from build123d import *

# Parameters (mm, degrees)
SKETCH_1_R      = 1
EXTRUDE_1_DEPTH = 1
FILLET_1_R      = 2


with BuildPart() as part:
    # 草图1 → 凸台-拉伸1 (new body)
    with BuildSketch(Plane(origin=(0, 0, 0), x_dir=(1, 0, 0), z_dir=(0, 1, 0))):
        with BuildLine():
            Line((20, 0), (16, 0))
            ThreePointArc((16, 0), (8, 13.856406461), (-8, 13.856406461))
            Line((-8, 13.856406461), (-10, 17.320508076))
            ThreePointArc((-10, 17.320508076), (10, 17.320508076), (20, 0))
        make_face()
        with Locations(Location((-4.658742812, 17.386664873, 0), (0, 0, 270))):
            Circle(SKETCH_1_R, mode=Mode.SUBTRACT)
        with Locations(Location((17.386664873, 4.658742812, 0), (0, 0, 270))):
            Circle(SKETCH_1_R, mode=Mode.SUBTRACT)
        with BuildLine():
            ThreePointArc((16.454482672, 9.5), (9.5, 16.454482672), (0, 19))
            ThreePointArc((0, 19), (-1, 18), (0, 17))
            ThreePointArc((0, 17), (8.5, 14.722431864), (14.722431864, 8.5))
            ThreePointArc((14.722431864, 8.5), (16.088457268, 8.133974596), (16.454482672, 9.5))
        make_face(mode=Mode.SUBTRACT)
    extrude(amount=EXTRUDE_1_DEPTH)

    # 圆角1
    fillet_1_edges = [part.edges().sort_by_distance(p)[0] for p in [
        (-8, 0.5, -13.856406461),
        (-10, 0.5, -17.320508076),
        (16, 0.5, 0),
        (20, 0.5, 0),
    ]]
    fillet(fillet_1_edges, radius=FILLET_1_R - 0.0001)  # a hair under: the kernel refuses the full size


solid = part.part
Read the model definition and answer for the solid it produces. Units are mm, in the model's axes. A direction names the side the tool comes from. Round coordinates to 2 decimals unless told otherwise and drop trailing zeros. Write each loop counter-clockwise with the first axis right and the second up, starting at its lowest first coordinate (ties: lowest second). Pieces come first, ordered by that corner, then holes. Notation, with made-up numbers: (39.25, -13) - (83.25, -13) arc R18 ccw to (83.25, 16) - close; hole circle Ø10 at (64, -35). An arc over 180 degrees is marked (long way). Use a Markdown table: item, result.
(1) The part is cut by section B-B (y = 0.6). State how many separate pieces and enclosed holes the cut face has, then the cut area to 3 significant figures.
Reported:
| item | result |
|---|---|
| separate pieces | 1 |
| enclosed holes | 3 |
| area | 100 mm2 |
(2) The mould has two halves that part along X. Classify faces 3 (the cylindrical face through (8.392, 0.493, -14.784)), 4 (the cylindrical face through (19.363, 0.507, -0.649)), 5 (the cylindrical face through (16.57, 0.507, -0.496)): released by +X, released by -X, zero draft, split by the parting line, or undercut.
Reported:
| item | result |
|---|---|
| face 3 | undercut |
| face 4 | released by +X |
| face 5 | released by -X |
(3) The part is cut by section A-A (z = -5). Write down the section's boundary in (x, y).
Reported:
| item | result |
|---|---|
| outline | (15.2, 0) - (16.45, 0) - (16.45, 1) - (15.2, 1) - close; (18.33, 0) - (19.36, 0) - (19.36, 1) - (18.33, 1) - close |
(4) Straight lines are drawn through the part: line 1 along Z through (x, y) = (2.25, 0.6); line 2 along X through (y, z) = (0.7, -11); line 3 along X through (y, z) = (0.4, -13). For each, find the intervals that lie inside material, in ascending order. Write a range as [from, to].
Reported:
| item | result |
|---|---|
| line 1 | [-19.87, -18.87], [-16.85, -15.84] |
| line 2 | [11.62, 12.96], [15.49, 16.7] |
| line 3 | [9.33, 10.95], [13.86, 15.2] |
(5) The part is cut by section C-C (x = -4). Write down the section's boundary in (y, z), then the cut area to 3 significant figures.
Reported:
| item | result |
|---|---|
| outline | (0, -19.6) - (1, -19.6) - (1, -18.14) - (0, -18.14) - close; (0, -16.63) - (1, -16.63) - (1, -15.49) - (0, -15.49) - close |
| area | 2.60 mm2 |
(6) The part is cut by section D-D (z = -18). Write down the section's boundary in (x, y), then the cut area to 3 significant figures.
Reported:
| item | result |
|---|---|
| outline | (-8.53, 0) - (-5.45, 0) - (-5.45, 1) - (-8.53, 1) - close; (-3.87, 0) - (-1, 0) - (-1, 1) - (-3.87, 1) - close; (6.08, 0) - (8.72, 0) - (8.72, 1) - (6.08, 1) - close |
| area | 8.58 mm2 |
(7) Which of the six approach directions +Z, -Z, +X, -X, +Y, -Y give full straight-line access (tool end or side, diameter ignored) to faces 1 (the cylindrical face through (-1, 0.5, -18)), 2 (the cylindrical face through (9.77, 0.49, -17.45))?
Reported:
| item | result |
|---|---|
| face 1 | +Y, -Y |
| face 2 | -Z, +Y, -Y |
